```python
from build123d import *

# Parameters (mm, degrees)
SKETCH_2_W           = 40.2
SKETCH_2_H           = 61.1
EXTRUDE_1_DEPTH      = 20.5
SKETCH_9_W           = 24.8
SKETCH_9_H           = 5.25
SKETCH_9_W_2         = 3.5
CUT_EXTRUDE_3_DEPTH  = 41.2
SKETCH_10_W          = 5.5
SKETCH_10_H          = 25
SKETCH_10_H_2        = 3.5
CUT_EXTRUDE_4_DEPTH  = 62.1
SKETCH_12_R          = 1.35
CUT_EXTRUDE_5_DEPTH  = 42
SKETCH_13_R          = 3.95
EXTRUDE_2_DEPTH      = 3.7
SKETCH_14_R          = 3.95
EXTRUDE_4_DEPTH      = 1
SKETCH_16_W          = 10.75
SKETCH_16_H          = 12.1
EXTRUDE_6_DEPTH      = 5.25
EXTRUDE_6_DEPTH_BACK = 34.25


with BuildPart() as part:
    # 스케치2 → 보스-돌출1 (new body, symmetric)
    with BuildSketch(Plane.XY):
        with Locations((20.1, 30.55)):
            Rectangle(SKETCH_2_W, SKETCH_2_H)
    extrude(amount=EXTRUDE_1_DEPTH, both=True)

    # 스케치9 → 컷-돌출3 (cut, through all)
    with BuildSketch(Plane(origin=(40.2, 0, 0), x_dir=(0, 0, -1), z_dir=(1, 0, 0))):
        with Locations((0, 2.625)):
            Rectangle(SKETCH_9_W, SKETCH_9_H)
        with Locations((-18.75, 2.625)):
            Rectangle(SKETCH_9_W_2, SKETCH_9_H)
        with Locations((18.75, 2.625)):
            Rectangle(SKETCH_9_W_2, SKETCH_9_H)
    extrude(amount=-CUT_EXTRUDE_3_DEPTH, mode=Mode.SUBTRACT)

    # 스케치10 → 컷-돌출4 (cut, through all)
    with BuildSketch(Plane(origin=(0, 61.1, 0), x_dir=(1, 0, 0), z_dir=(0, 1, 0))):
        with Locations((2.75, 0)):
            Rectangle(SKETCH_10_W, SKETCH_10_H)
        with Locations((2.75, 18.75)):
            Rectangle(SKETCH_10_W, SKETCH_10_H_2)
        with Locations((37.45, 0)):
            Rectangle(SKETCH_10_W, SKETCH_10_H)
        with Locations((37.45, 18.75)):
            Rectangle(SKETCH_10_W, SKETCH_10_H_2)
        with Locations((2.75, -18.75)):
            Rectangle(SKETCH_10_W, SKETCH_10_H_2)
        with Locations((37.45, -18.75)):
            Rectangle(SKETCH_10_W, SKETCH_10_H_2)
    extrude(amount=-CUT_EXTRUDE_4_DEPTH, mode=Mode.SUBTRACT)

    # 스케치12 → 컷-돌출5 (cut, through all)
    with BuildSketch(Plane.XY.offset(20.5)):
        with Locations((9.1, 2.8)):
            Circle(SKETCH_12_R)
        with Locations((31.1, 2.8)):
            Circle(SKETCH_12_R)
        with Locations((2.8, 52.1)):
            Circle(SKETCH_12_R)
        with Locations((37.4, 52.1)):
            Circle(SKETCH_12_R)
        with Locations((2.8, 30.1)):
            Circle(SKETCH_12_R)
        with Locations((37.4, 30.1)):
            Circle(SKETCH_12_R)
        with Locations((2.8, 8.1)):
            Circle(SKETCH_12_R)
        with Locations((37.4, 8.1)):
            Circle(SKETCH_12_R)
    extrude(amount=-CUT_EXTRUDE_5_DEPTH, mode=Mode.SUBTRACT)

    # 스케치13 → 보스-돌출2 (add)
    with BuildSketch(Plane.XY.offset(20.5)):
        with Locations((20.1, 48.1)):
            Circle(SKETCH_13_R)
    extrude(amount=EXTRUDE_2_DEPTH)

    # 스케치14 → 보스-돌출4 (add)
    with BuildSketch(Plane(origin=(0, 0, -20.5), x_dir=(-1, 0, 0), z_dir=(0, 0, -1))):
        with Locations((-20.1, 48.1)):
            Circle(SKETCH_14_R)
    extrude(amount=EXTRUDE_4_DEPTH)

    # 스케치16 → 보스-돌출6 (add, two sides)
    with BuildSketch(Plane(origin=(34.7, 0, 0), x_dir=(0, 0, -1), z_dir=(1, 0, 0))) as extrude_6_sk:
        with Locations((7.125, 16.8)):
            Rectangle(SKETCH_16_W, SKETCH_16_H)
    extrude(amount=EXTRUDE_6_DEPTH)
    extrude(extrude_6_sk.sketch, amount=-EXTRUDE_6_DEPTH_BACK)


solid = part.part
```
Part model, mm, in its own coordinate system. A direction names the side the tool comes from. Give positions to 0.01 mm unless a question says otherwise; leave off trailing zeros. Order: outer loops, then holes, each group sorted by start corner. A loop starts at its lowest first (then second) coordinate and runs counter-clockwise, first axis right, second up. Notation, with made-up numbers: (1, 6.25) - (45, 6.25) arc R27 cw to (45, 38.25) - close; hole circle Ø8 at (71, -35). An arc over 180 degrees is marked (long way). Use one line per item in the form item = value.
Item 1: Slice it at A-A on x = 9.1. Give the cut face in (y, z), and give its area (3 significant figures).
Solution:
outline = (0, -17) - (1.45, -17) - (1.45, -12.4) - (0, -12.4) - close; (0, 12.4) - (1.45, 12.4) - (1.45, 17) - (0, 17) - close; (4.15, -17) - (5.25, -17) - (5.25, -20.5) - (61.1, -20.5) - (61.1, 20.5) - (5.25, 20.5) - (5.25, 17) - (4.15, 17) - (4.15, 12.4) - (5.25, 12.4) - (5.25, -12.4) - (4.15, -12.4) - close
area = 2,310 mm2
Item 2: Two-plate mould, pull along Y, no slides. Class faces 5 (the face through (20, 61.1, 0)), 6 (the face through (38.688, 30.506, -14.718)), 7 (the face through (0, 30, -15)): released by +Y, released by -Y, zero draft, split by the parting line, or undercut.
Solution:
face_5 = released by +Y
face_6 = undercut
face_7 = zero draft
Item 3: Probe probe 1 along X at (y, z) = (8, -14); probe 2 along Y at (x, z) = (2.8, -14.5); probe 3 along Y at (x, z) = (2, -15). List the from-to ranges inside material, lowest first. Write a range as from..to.
Solution:
probe_1 = 0..1.45, 4.15..36.05, 38.75..40.2
probe_2 = 0..6.75, 9.45..28.75, 31.45..50.75, 53.45..61.1
probe_3 = 0..7.01, 9.19..29.01, 31.19..51.01, 53.19..61.1
Item 4: Which spindle directions (+Z, -Z, +X, -X, +Y, -Y) get a long thin tool onto all of the face, cutting with end or side? Do faces 1 (the face through (1, 31, -12.5)), 2 (the face through (39.95, 17, -7)), 3 (the face through (34.7, 34, 19)), 4 (the face through (5.5, 34, 19)). Say none if no direction does.
Solution:
face_1 = -X
face_2 = +X, +Y, -Y
face_3 = +Z, +X, +Y, -Y
face_4 = +Z, -X, +Y, -Y
Item 5: Slice it at B-B on y = 27. Give the cut face in (x, z), and give its area (3 significant figures).
Solution:
outline = (0, -17) - (5.5, -17) - (5.5, -20.5) - (34.7, -20.5) - (34.7, -17) - (40.2, -17) - (40.2, -12.5) - (34.7, -12.5) - (34.7, 12.5) - (40.2, 12.5) - (40.2, 17) - (34.7, 17) - (34.7, 20.5) - (5.5, 20.5) - (5.5, 17) - (0, 17) - (0, 12.5) - (5.5, 12.5) - (5.5, -12.5) - (0, -12.5) - close
area = 1,300 mm2
Item 6: Pin check, flat tips, straight feed: pin 1 Ø3.5 at (x, y) = (2.8, 8.1) entering from -Z; pin 2 Ø4 at (x, z) = (37.5, -7) entering from +Y; pin 3 Ø4 at (x, y) = (15, 4) entering from -Z; pin 4 Ø10 at (y, z) = (30, 9.5) entering from +X. Stop position of each tip, or through.
Solution:
pin_1 = -17
pin_2 = 22.85
pin_3 = -20.5
pin_4 = 40.2
Item 7: Slice it at C-C on z = 15. Count the separate pieces of the cut face and the enclosed holes in it, and give its area (3 significant figures).
Solution:
separate_pieces = 1
enclosed_holes = 8
area = 2,410 mm2
Item 8: Slice it at D-D on x = 25. Give the cut face in (y, z).
Solution:
outline = (0, -17) - (5.25, -17) - (5.25, -20.5) - (61.1, -20.5) - (61.1, 20.5) - (5.25, 20.5) - (5.25, 17) - (0, 17) - (0, 12.4) - (5.25, 12.4) - (5.25, -12.4) - (0, -12.4) - close
